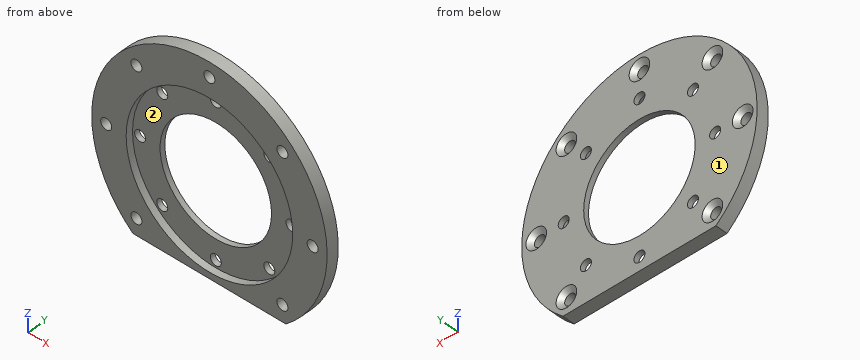
from build123d import *

# Parameters (mm, degrees)
ESQUISSE3_R                                    = 1.6
ENL_V_MAT_EXTRU_1_DEPTH                        = 4.5
FRAISAGE_POUR_VIS_T_TE_FRAIS_E_100_D           = 3.2
FRAISAGE_POUR_VIS_T_TE_FRAIS_E_100_CSINK_D     = 6
FRAISAGE_POUR_VIS_T_TE_FRAIS_E_100_CSINK_ANGLE = 100
R_P_TITION_CIRCULAIRE1_COUNT                   = 8
SKETCH1_W                                      = 44.436021424
SKETCH1_H                                      = 8.2
CUT_EXTRUDE1_DEPTH                             = 4.5


with BuildPart() as part:
    # Esquisse2 → Révolution1 (revolve)
    with BuildSketch(Plane.XY):
        Polygon((34.2, 0), (34.2, 3.5), (16.2, 3.5), (16.2, 2), (24.2, 2), (24.2, 0), align=None)
    revolve(axis=Axis((0, 37.373365456, 0), (0, -1, 0)))

    # Esquisse3 → Enlèv. mat.-Extru.1 (cut, through all)
    with BuildSketch(Plane(origin=(0, 3.5, 0), x_dir=(1, 0, 0), z_dir=(0, 1, 0))):
        with Locations((22, 0)):
            Circle(ESQUISSE3_R)
    enl_v_mat_extru_1 = extrude(amount=-ENL_V_MAT_EXTRU_1_DEPTH, mode=Mode.SUBTRACT)

    # Fraisage pour vis à tête fraisée (100) #01 (through all)
    with Locations(Plane(origin=(0, 3.5, 0), x_dir=(1, 0, 0), z_dir=(0, 1, 0))):
        with Locations((30, 0)):
            fraisage_pour_vis_t_te_frais_e_100 = CounterSinkHole(FRAISAGE_POUR_VIS_T_TE_FRAIS_E_100_D / 2, FRAISAGE_POUR_VIS_T_TE_FRAIS_E_100_CSINK_D / 2, counter_sink_angle=FRAISAGE_POUR_VIS_T_TE_FRAIS_E_100_CSINK_ANGLE)

    # Répétition circulaire1: Enlèv. mat.-Extru.1, Fraisage pour vis à tête fraisée (100) #01 ×8 about axis
    r_p_tition_circulaire1_axis = Axis((0, 0, 0), (0, 1, 0))
    for i in range(1, R_P_TITION_CIRCULAIRE1_COUNT):
        add(enl_v_mat_extru_1.rotate(r_p_tition_circulaire1_axis, i * 360 / R_P_TITION_CIRCULAIRE1_COUNT), mode=Mode.SUBTRACT)
        add(fraisage_pour_vis_t_te_frais_e_100.rotate(r_p_tition_circulaire1_axis, i * 360 / R_P_TITION_CIRCULAIRE1_COUNT), mode=Mode.SUBTRACT)

    # Sketch1 → Cut-Extrude1 (cut, through all)
    with BuildSketch(Plane(origin=(0, 0, 0), x_dir=(-1, 0, 0), z_dir=(0, -1, 0))):
        with Locations((0, 30.1)):
            Rectangle(SKETCH1_W, SKETCH1_H)
    extrude(amount=-CUT_EXTRUDE1_DEPTH, mode=Mode.SUBTRACT)


solid = part.part
The listing builds one solid part. Answer for the finished solid, in the listing's coordinates (mm). Face numbers are marked on the shaded views. Give positions to 0.01 mm unless a question says otherwise; leave off trailing zeros. Order: outer loops, then holes, each group sorted by start corner. A loop starts at its lowest first (then second) coordinate and runs counter-clockwise, first axis right, second up. Notation, with made-up numbers: (63.5, 63.5) - (69.5, 63.5) arc R34 ccw to (69.5, 102.5) - close; hole circle Ø6 at (45, -7). An arc over 180 degrees is marked (long way). One line per item, written item: value. Start each with the question number.
1) A cutting plane is placed at D-D on z = -6.5. Give the vertices of the cut face in (x, y), then the cut area to 3 significant figures.
2) Given pin 1 Ø5 at (x, z) = (30, 0) entering from +Y; pin 2 Ø3 at (x, z) = (22, 0) entering from -Y; pin 3 Ø2 at (y, z) = (2, 18) entering from +X; pin 4 Ø2 at (x, y) = (25.5, 1) entering from +Z, each flat-ended and moving along its own axis, determine where each tip first touches the part or whether it passes through.
3) A cutting plane is placed at B-B on z = 0. State how many separate pieces and enclosed holes the cut face has, then the cut area to 3 significant figures.
4) Find the intervals of material crossed by L1, parallel to X at y = 2.7, z = -17; L2, parallel to X at y = 1.75, z = 20; L3, parallel to Y at x = 10.5, z = -18.5, in increasing order.
5) The mould has two halves that part along X. Classify the marked faces 1 and 2: released by +X, released by -X, zero draft, split by the parting line, or undercut.
6) A cutting plane is placed at A-A on x = 0. Give the vertices of the cut face in (y, z).
Answer sheet:
1. outline: (-33.58, 0) - (-23.31, 0) - (-23.31, 2) - (-14.84, 2) - (-14.84, 3.5) - (-33.58, 3.5) - close; (14.84, 2) - (23.31, 2) - (23.31, 0) - (33.58, 0) - (33.58, 3.5) - (14.84, 3.5) - close
1. area: 97.3 mm2
2. pin 1: stops at y = 3.08
2. pin 2: passes through
2. pin 3: stops at x = 29.68
2. pin 4: stops at z = 23.86
3. separate pieces: 6
3. enclosed holes: 0
3. area: 58.7 mm2
4. L1: x = -29.68 to -16.25, -14.87 to 14.87, 16.25 to 29.68
4. L2: x = -27.74 to -22.26, -20.17 to -13.62, 13.62 to 20.17, 22.26 to 27.74
4. L3: y = 2 to 3.5
5. face 1: zero draft
5. face 2: undercut
6. outline: (0, -26) - (3.5, -26) - (3.5, -23.6) - (2, -23.6) - (2, -24.2) - (0, -24.2) - close; (0, 24.2) - (2, 24.2) - (2, 23.6) - (3.5, 23.6) - (3.5, 27) - (2.33, 28.4) - (0, 28.4) - close; (0, 31.6) - (2.33, 31.6) - (3.5, 33) - (3.5, 34.2) - (0, 34.2) - close; (2, -20.4) - (3.5, -20.4) - (3.5, -16.2) - (2, -16.2) - close; (2, 16.2) - (3.5, 16.2) - (3.5, 20.4) - (2, 20.4) - close
